Check sheet for the modelled part. Datum: model origin and axes. Units: mm. A direction names the side the tool comes from. Round coordinates to 2 decimals unless told otherwise and drop trailing zeros. Loops run counter-clockwise (first coordinate to the right, second up) from the corner with the lowest first, then second, coordinate; pieces in that order, holes last. Notation, with made-up numbers: (24.25, 62.25) -> (62.25, 62.25) arc R21 ccw to (62.25, 75.25) -> close; hole circle Ø8 at (-25, -26). An arc over 180 degrees is marked (long way). One line per question, with ' | ' between items.
```python
from build123d import *

# Parameters (mm, degrees)
F0_R        = 40
F0_R_2      = 25
F1_DEPTH    = 10
F0_R_3      = 20
F2_DEPTH    = 20
F0_R_4      = 7.5
F3_DEPTH    = 135
F4_DEPTH    = 160
F5_S8_R     = 20
F5_T9_DEPTH = 37
F6_SIZE2    = 3
F6_SIZE     = 3


# Not quite as in the source:
# - a fillet or chamfer that OpenCascade refuses, or shapes differently, is made with other operations: its cross-section is extruded or revolved along the edge and cut away or added


with BuildPart() as f1:
    # F0 (on Right) → F1 (new body)
    with BuildSketch(Plane.YZ):
        Circle(F0_R)
        Circle(F0_R_2, mode=Mode.SUBTRACT)
    extrude(amount=-F1_DEPTH)

    # F0 (on Right) → F2 (join)
    with BuildSketch(Plane.YZ):
        Circle(F0_R_2)
        Circle(F0_R_3, mode=Mode.SUBTRACT)
    extrude(amount=-F2_DEPTH)

    # F0 (on Right) → F3 (join)
    with BuildSketch(Plane.YZ):
        Circle(F0_R_3)
        Circle(F0_R_4, mode=Mode.SUBTRACT)
    extrude(amount=-F3_DEPTH)

    # F0 (on Right) → F4 (join)
    with BuildSketch(Plane.YZ):
        Circle(F0_R_4)
    extrude(amount=-F4_DEPTH)

    # F5: chamfer of 10 on 2 edges, made by hand

    # F5_s1 → F5_t2 (revolve, cut)
    with BuildSketch(Plane.XY):
        Polygon((-10, 40), (0, 30), (0, 40), align=None)
    revolve(axis=Axis((0, 0, 0), (1, 0, 0)), mode=Mode.SUBTRACT)


with BuildPart() as f5_tool4:
    # F5_s5 → F5_t6 (revolve)
    with BuildSketch(Plane.XY):
        Polygon((-10, 25), (-20, 15), (-20, 25), align=None)
    revolve(axis=Axis((-20, 0, 0), (1, 0, 0)))

    split(bisect_by=Plane.YZ.offset(-10), keep=Keep.BOTTOM)

    # F5_s8 → F5_t9 (cut, symmetric)
    with BuildSketch(Plane.YZ.offset(-15)):
        Circle(F5_S8_R)
    extrude(amount=F5_T9_DEPTH, both=True, mode=Mode.SUBTRACT)


with BuildPart() as f1_1:
    add(f1.part)

    # F5_t3: cut F5_tool4
    add(f5_tool4.part, mode=Mode.SUBTRACT)

    # F6
    f6_edges = [f1_1.edges().sort_by_distance(p)[0] for p in [
        (-135, -20, 0),
    ]]
    chamfer(f6_edges, length=F6_SIZE, length2=F6_SIZE2)


solid = f1_1.part
```
(1) Set-up check for faces 1 (the face through (-72.681, -4.336, -19.524)), 2 (the face through (0, 0, 0)): record each of +Z, -Z, +X, -X, +Y, -Y from which the full face is reachable in a straight line by a thin tool's end or side.
Answer:
face 1: -X | face 2: +Z, -Z, +X, +Y, -Y
(2) Scan lines: probe 1 along X at (y, z) = (-4, -8.5); probe 2 along X at (y, z) = (-20, -24.5); probe 3 along Z at (x, y) = (-65.5, -1.5). Record each from-to range of solid material in increasing order.
Answer:
probe 1: x = -135 to 0 | probe 2: x = -10 to -1.63 | probe 3: z = -19.94 to 19.94
(3) Sectioned sample at D-D, the plane x = -139. Record the cut outline in (y, z), and give its area (3 significant figures).
Answer:
outline: circle Ø15 at (0, 0) | area: 177 mm2
(4) Sectioned sample at C-C, the plane x = -32.5. Record the cut outline in (y, z), and give its area (3 significant figures).
Answer:
outline: circle Ø40 at (0, 0) | area: 1,260 mm2
(5) Sectioned sample at A-A, the plane y = 0. Record the cut outline in (x, z), and give its area (3 significant figures).
Answer:
outline: (-160, -7.5) -> (-135, -7.5) -> (-135, -17) -> (-132, -20) -> (-15, -20) -> (-10, -25) -> (-10, -40) -> (0, -30) -> (0, 30) -> (-10, 40) -> (-10, 25) -> (-15, 20) -> (-132, 20) -> (-135, 17) -> (-135, 7.5) -> (-160, 7.5) -> close | area: 6,090 mm2
(6) Go/stop test with flat-tipped pins: pin 1 (2 mm diameter, centred on x = -133, y = -16, fed in from -Z); pin 2 (8 mm diameter, centred on x = -116.5, z = 16, fed in from -Y); pin 3 (10 mm diameter, centred on x = -92, z = -22.5, fed in from -Y); pin 4 (5 mm diameter, centred on y = 8, z = -26.5, fed in from +X). Record where each tip stops, or that it passes through.
Answer:
pin 1: stops at z = -12.45 | pin 2: stops at y = -16 | pin 3: stops at y = -9.68 | pin 4: stops at x = 0
